Autodesk Fusion 360 part; units mm, degrees
sketch "Sketch1" plane through (0, 0, 0) normal (1, 0, 0) x (0, 1, 0)
  line L0 (-19.1488, 16.2315) -> (19.1512, 16.2315)
  line L1 (19.1512, 16.2315) -> (19.1512, -16.3685)
  line L2 (19.1512, -16.3685) -> (-19.1488, -16.3685)
  line L3 (-19.1488, -16.3685) -> (-19.1488, 16.2315)
  circle A0 centre (-15.3988, -0.9685) radius 1.1
  circle A1 centre (15.4012, 6.9815) radius 1.1
  circle A2 centre (9.1512, -12.8825) radius 1.1
  line L4 (19.1512, -9.8685) -> (11.6512, -9.8685)
  line L5 (11.6512, -9.8685) -> (11.6512, -1.5685)
  line L6 (11.6512, -1.5685) -> (19.1512, -1.5685)
  line L7 (19.1512, -1.5685) -> (19.1512, -9.8685)
  dimension "d1" = 38.3
  dimension "d2" = 32.6
  dimension "d3" = 2.2
  dimension "d4" = 15.4
  dimension "d5" = 3.75
  dimension "d6" = 2.2
  dimension "d7" = 9.25
  dimension "d8" = 3.75
  dimension "d9" = 2.2
  dimension "d10" = 10
  dimension "d11" = 3.486
  dimension "d23" = 7.5
  dimension "d24" = 8.3
  dimension "d25" = 6.5
extrude "Extrude1" add sketch "Sketch1" along normal blind 3
sketch "Sketch2" plane through (3, 0, 0) normal (1, 0, 0) x (0, 1, 0)
  circle A0 centre (9.1512, -12.8825) radius 1.1
  circle A1 centre (15.4012, 6.9815) radius 1.1
  circle A2 centre (-15.3988, -0.9685) radius 1.1
  line L0 (-19.1488, -16.3685) -> (19.1512, -16.3685)
  line L1 (19.1512, -16.3685) -> (19.1512, 16.2315)
  line L2 (19.1512, 16.2315) -> (-19.1488, 16.2315)
  line L3 (-19.1488, 16.2315) -> (-19.1488, -16.3685)
  circle A3 centre (-15.3988, -0.9685) radius 2.4
  circle A4 centre (9.1512, -12.8825) radius 2.4
  circle A5 centre (15.4012, 6.9815) radius 2.4
  dimension "d14" = 4.8
  dimension "d15" = 4.8
  dimension "d16" = 4.8
extrude "Extrude2" cut sketch "Sketch2" against normal blind 1.5 contours A3
extrude "Extrude3" cut sketch "Sketch2" against normal blind 1.5 contours A4
extrude "Extrude4" cut sketch "Sketch2" against normal blind 1.5 contours A5
extrude "Extrude5" cut sketch "Sketch1" along normal blind 3 contours L1 L4 L5 L6 L7
fillet "Fillet1" radius 1 1 edges at (3, 0.0012, 16.2315)
fillet "Fillet2" radius 1 3 edges at (1, -19.1488, 16.2315) (2.7071, -19.1488, 15.9387) (3, -19.1488, -0.5685)
fillet "Fillet3" radius 1 3 edges at (1, -19.1488, -16.3685) (2.7071, -18.856, -16.3685) (3, 0.5012, -16.3685)
fillet "Fillet4" radius 1 3 edges at (1, 19.1512, -16.3685) (2.7071, 19.1512, -16.0756) (3, 19.1512, -12.6185)
fillet "Fillet5" radius 1 3 edges at (1, 19.1512, -9.8685) (2.7071, 18.8583, -9.8685) (3, 14.9012, -9.8685)
fillet "Fillet6" radius 1 1 edges at (3, 11.6512, -6.2185)
fillet "Fillet7" radius 1 1 edges at (3, 14.9012, -1.5685)
fillet "Fillet8" radius 1 5 edges at (1, 19.1512, -1.5685) (2.7071, 19.1512, -1.2756) (3, 19.1512, 7.3315) (2.7071, 19.1512, 15.9387) (1, 19.1512, 16.2315)
Geometry: final body of the model. Coordinates: model frame, mm. A direction names the side the tool comes from. Coordinates: 2 decimals unless noted, no trailing zeros. Order: outer loops, then holes, each group sorted by start corner. A loop starts at its lowest first (then second) coordinate and runs counter-clockwise, first axis right, second up. Notation, with made-up numbers: (84, 67) - (113, 67) arc R8 cw to (113, 74) - close; hole circle Ø5 at (1, 22.5). An arc over 180 degrees is marked (long way). Use one line per item in the form item = value.
1) Section B-B (x = 0.95). Return loops of the section in (y, z), then the cut area to 3 significant figures.
Solutions:
outline = (-19.15, -15.37) arc R1 ccw to (-18.15, -16.37) - (18.15, -16.37) arc R1 ccw to (19.15, -15.37) - (19.15, -10.87) arc R1 ccw to (18.15, -9.87) - (11.65, -9.87) - (11.65, -1.57) - (18.15, -1.57) arc R1 ccw to (19.15, -0.57) - (19.15, 15.23) arc R1 ccw to (18.15, 16.23) - (-18.15, 16.23) arc R1 ccw to (-19.15, 15.23) - close; hole circle Ø2.2 at (-15.4, -0.97); hole circle Ø2.2 at (9.15, -12.88); hole circle Ø2.2 at (15.4, 6.98)
area = 1,170 mm^2
2) Set-up query: faces 1 (the face through (1.014, 18.85, -16.083)), 2 (the face through (1, 0, 16.232)), 3 (the face through (2.699, 11.366, -5.791)), 4 (the face through (1.5, -14, -1)), 5 (the face through (1, 11.651, -6)). Return all of +Z, -Z, +X, -X, +Y, -Y with unobstructed straight access to the full face (end or side cutting, diameter ignored); none if empty.
Solutions:
face_1 = -Z, +X, -X, +Y
face_2 = +Z, +X, -X, +Y, -Y
face_3 = +X, +Y
face_4 = +X
face_5 = +X, -X, +Y
3) Section C-C (z = -9). Return loops of the section in (x, y).
Solutions:
outline = (0, -19.15) - (2, -19.15) arc R1 ccw to (3, -18.15) - (3, 10.65) arc R1 ccw to (2, 11.65) - (0, 11.65) - close
4) Section D-D (y = 7.5). Return loops of the section in (x, z), then the cut area to 3 significant figures.
Solutions:
outline = (0, -16.37) - (2, -16.37) arc R1 ccw to (3, -15.37) - (3, -14.62) - (1.5, -14.62) - (1.5, -11.14) - (3, -11.14) - (3, 15.23) arc R1 ccw to (2, 16.23) - (0, 16.23) - close
area = 92.1 mm^2
5) Pin query (flat end, axial travel): pin 1 (1.8 mm diameter, centred on y = -15.4, z = -0.97, fed in from +X); pin 2 (0.6 mm diameter, centred on x = 1.5, z = -5, fed in from +Y); pin 3 (3 mm diameter, centred on y = 15.4, z = 6.98, fed in from +X). Return the tip coordinate at first contact, or that it passes through.
Solutions:
pin_1 = through
pin_2 = 11.65
pin_3 = 1.5
6) Ray query, L1, parallel to Z at x = 0.25, y = 15.5; L2, parallel to Z at x = 1.15, y = 13.5; L3, parallel to Y at x = 0.8, z = -12.5. Return the intervals inside material, ascending.
Solutions:
L1 = -16.37 to -9.87, -1.57 to 5.89, 8.08 to 16.23
L2 = -16.37 to -9.87, -1.57 to 16.23
L3 = -19.15 to 8.12, 10.18 to 19.15
7) Section A-A (y = -15.5). Return loops of the section in (x, z), then the cut area to 3 significant figures.
Solutions:
outline = (0, -16.37) - (2, -16.37) arc R1 ccw to (3, -15.37) - (3, -3.37) - (1.5, -3.37) - (1.5, -2.06) - (0, -2.06) - close; (0, 0.13) - (1.5, 0.13) - (1.5, 1.43) - (3, 1.43) - (3, 15.23) arc R1 ccw to (2, 16.23) - (0, 16.23) - close
area = 86.9 mm^2
